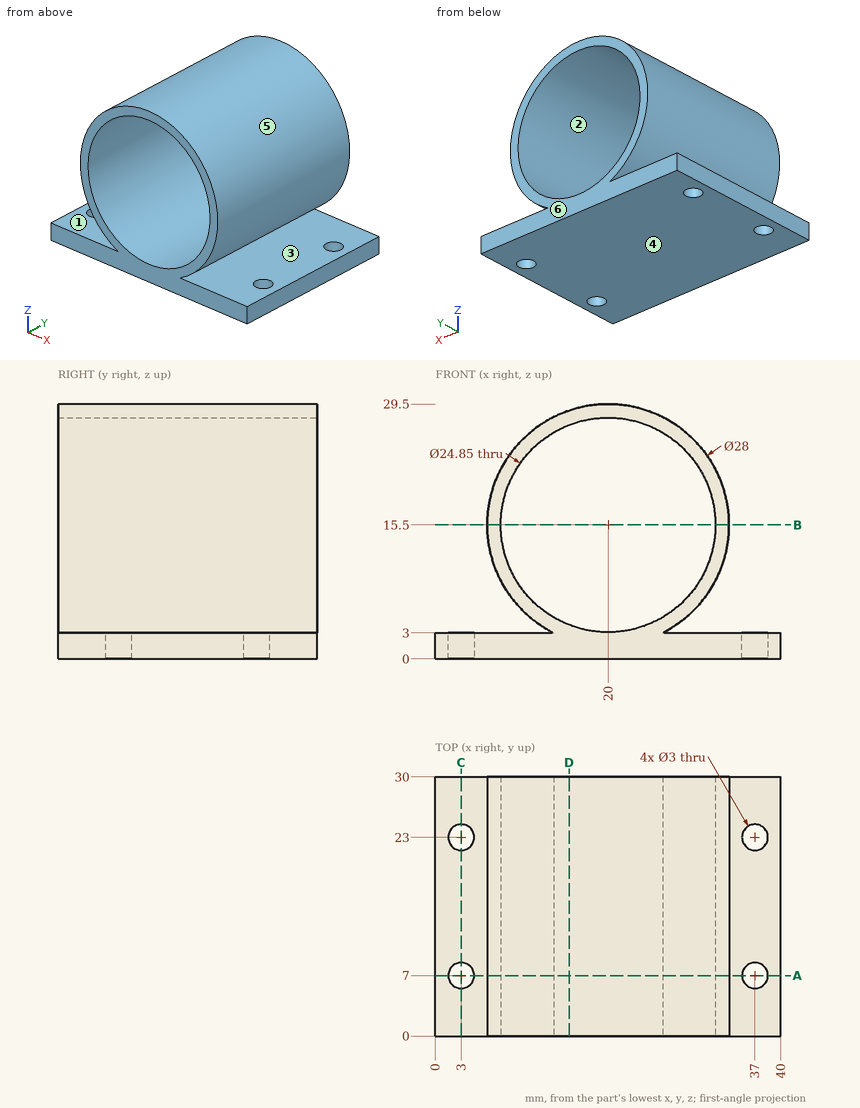
The drawing under review shows one solid part. Ordinate dimensions are in mm from its lowest x, y, z. A direction names the side the tool comes from. Give positions to 0.01 mm unless a question says otherwise; leave off trailing zeros. Order: outer loops, then holes, each group sorted by start corner. A loop starts at its lowest first (then second) coordinate and runs counter-clockwise, first axis right, second up. Notation, with made-up numbers: M 89,59.5 L 104,59.5 A15 ccw 104,86.5 Z; hole C 25.25,6.5 d2. An arc over 180 degrees is marked long. Answer in a Markdown table with one row per item. Add a question column.
1. To check wall thickness, follow line 1 along Y through (x, z) = (3, 1.3); line 2 along Z through (x, y) = (20.5, 6); line 3 along Z through (x, y) = (31, 24.5). State the ranges of each line that lie inside material, in increasing order.
2. Add section A-A on y = 7. State the section outline as (x, z) points (3 decimals).
3. Add section D-D on x = 15.5. State the section outline as (y, z) points.
4. Add section B-B on z = 15.5. State the section outline as (x, y) points (3 decimals), plus the area to 3 significant figures.
5. Add section C-C on x = 3. State the section outline as (y, z) points, plus the area to 3 significant figures.
6. For pin 1 Ø6 at (x, y) = (31, 18.5) entering from +Z; pin 2 Ø6 at (y, z) = (11.5, 12) entering from -X; pin 3 Ø12 at (y, z) = (25.5, 5.5) entering from -X; pin 4 Ø12 at (x, z) = (15, 14) entering from -Y, all flat-tipped, find the tip position at first contact; note any pin that passes through.
7. Machinability: for the marked faces 1, 2 and 3, which of the approach directions +Z, -Z, +X, -X, +Y, -Y give a long, thin tool a straight path to every point of the face, cutting with its end or side? Answer none if there is none.
8. Mouldability with a two-part tool opening along Z and no side actions: class the marked faces 4, 5 and 6 as released by +Z, released by -Z, zero draft, split by the parting line, or undercut.
The answers:
| question | item | result |
|---|---|---|
| 1 | line 1 | 0 to 5.5, 8.5 to 21.5, 24.5 to 30 |
| 1 | line 2 | 0 to 3.09, 27.91 to 29.49 |
| 1 | line 3 | 0 to 3, 6.84 to 9.72, 21.28 to 24.16 |
| 2 | outline | M 0,0 L 1.5,0 L 1.5,3 L 0,3 Z; M 4.5,0 L 35.5,0 L 35.5,3 L 26.305,3 A14 ccw long 13.695,3 L 4.5,3 Z; M 38.5,0 L 40,0 L 40,3 L 38.5,3 Z; hole C 20,15.5 d24.85 |
| 3 | outline | M 0,0 L 30,0 L 30,3.92 L 0,3.92 Z; M 0,27.08 L 30,27.08 L 30,28.76 L 0,28.76 Z |
| 4 | outline | M 6,0 L 7.575,0 L 7.575,30 L 6,30 Z; M 32.425,0 L 34,0 L 34,30 L 32.425,30 Z |
| 4 | area | 94.5 mm2 |
| 5 | outline | M 0,0 L 5.5,0 L 5.5,3 L 0,3 Z; M 8.5,0 L 21.5,0 L 21.5,3 L 8.5,3 Z; M 24.5,0 L 30,0 L 30,3 L 24.5,3 Z |
| 5 | area | 72.0 mm2 |
| 6 | pin 1 | z = 26.99 |
| 6 | pin 2 | x = 6.01 |
| 6 | pin 3 | x = 0 |
| 6 | pin 4 | through |
| 7 | face 1 | -X, +Y, -Y |
| 7 | face 2 | +Y, -Y |
| 7 | face 3 | +X, +Y, -Y |
| 8 | face 4 | released by -Z |
| 8 | face 5 | undercut |
| 8 | face 6 | zero draft |
